The figure shows three views and two pictorial views of one solid part (mm, origin at its lowest corner). Answer the questions. Round coordinates to 2 decimals unless told otherwise and drop trailing zeros. Write each loop counter-clockwise with the first axis right and the second up, starting at its lowest first coordinate (ties: lowest second). Pieces come first, ordered by that corner, then holes. Notation, with made-up numbers: (65.25, 15) - (109.25, 15) arc R32 cw to (109.25, 48) - close; hole circle Ø2 at (63, 80). An arc over 180 degrees is marked (long way). Answer as CSV lines item,"result". Start each with the question number.
Item 1: A cutting plane is placed at B-B on z = 3.2. Determine the outline of the cut face in (x, y) (1 decimal), and give its area (3 significant figures).
Item 2: A cutting plane is placed at C-C on x = 17. Determine the outline of the cut face in (y, z), and give its area (3 significant figures).
Item 3: For a pull along X with two mould halves and no side action, classify the marked faces 1, 2, 3 and 4 as pulls with the +X half, pulls with the -X half, needs draft (parallel to the pull), parting line crosses it, or undercut.
Item 4: A flat-ended cylindrical pin translates along its axis: pin 1 (6 mm diameter, centred on x = 31.5, y = 41.5, fed in from -Z). Find the tip coordinate at first contact, or state that the pin passes through.
Item 5: A cutting plane is placed at D-D on x = 26.5. Determine the outline of the cut face in (y, z) (3 decimals).
Item 6: A cutting plane is placed at A-A on y = 10. Determine the outline of the cut face in (x, z), and give its area (3 significant figures).
Item 7: Straight lines are drawn through the part: line 1 along X through (y, z) = (28.5, 1.65); line 2 along X through (y, z) = (39, 2.4); line 3 along Y through (x, z) = (16.5, 1.2). For each, find the intervals that lie inside material, in ascending order. Write a range as [from, to].
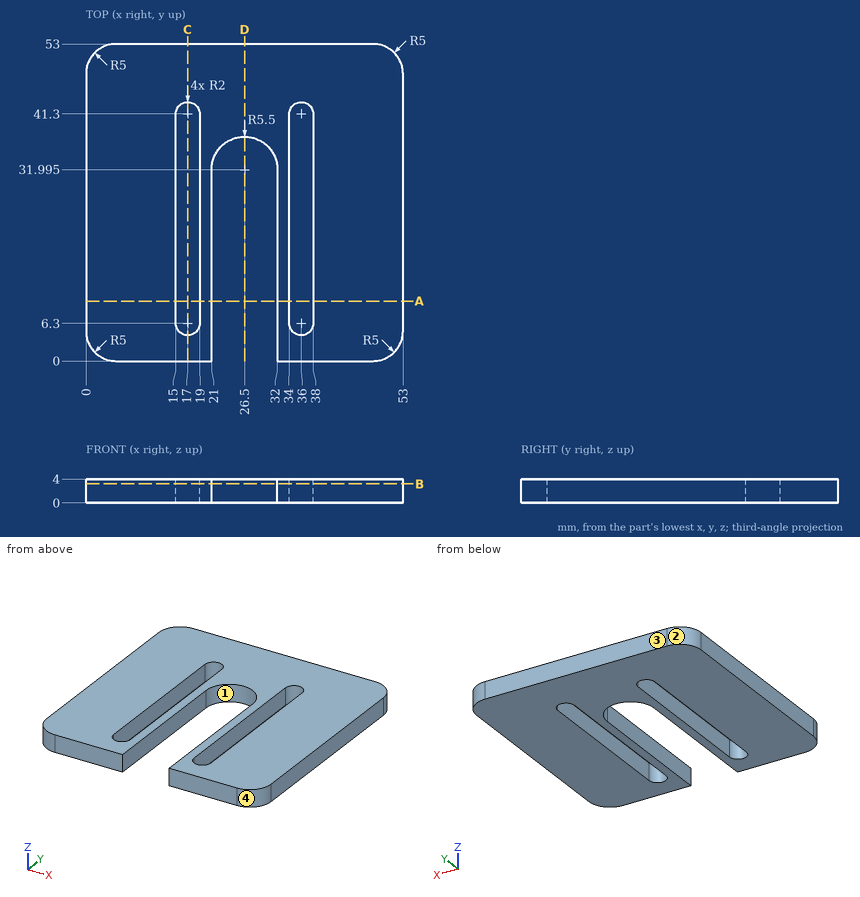
Geometry says:
1,outline,"(0, 5) arc R5 ccw to (5, 0) - (21, 0) - (21, 32) arc R5.5 cw to (32, 32) - (32, 0) - (48, 0) arc R5 ccw to (53, 5) - (53, 48) arc R5 ccw to (48, 53) - (5, 53) arc R5 ccw to (0, 48) - close; hole (15, 6.3) arc R2 ccw to (19, 6.3) - (19, 41.3) arc R2 ccw to (15, 41.3) - close; hole (34, 6.3) arc R2 ccw to (38, 6.3) - (38, 41.3) arc R2 ccw to (34, 41.3) - close"
1,area,"2,080 mm^2"
2,outline,"(0, 0) - (4.3, 0) - (4.3, 4) - (0, 4) - close; (43.3, 0) - (53, 0) - (53, 4) - (43.3, 4) - close"
2,area,"56.0 mm^2"
3,face 1,"undercut"
3,face 2,"pulls with the -X half"
3,face 3,"needs draft"
3,face 4,"pulls with the +X half"
4,pin 1,"stops at z = 0"
5,outline,"(37.495, 0) - (53, 0) - (53, 4) - (37.495, 4) - close"
6,outline,"(0, 0) - (15, 0) - (15, 4) - (0, 4) - close; (19, 0) - (21, 0) - (21, 4) - (19, 4) - close; (32, 0) - (34, 0) - (34, 4) - (32, 4) - close; (38, 0) - (53, 0) - (53, 4) - (38, 4) - close"
6,area,"136 mm^2"
7,line 1,"x = [0, 15], [19, 21], [32, 34], [38, 53]"
7,line 2,"x = [0, 15], [19, 34], [38, 53]"
7,line 3,"y = [0, 4.36], [43.24, 53]"
